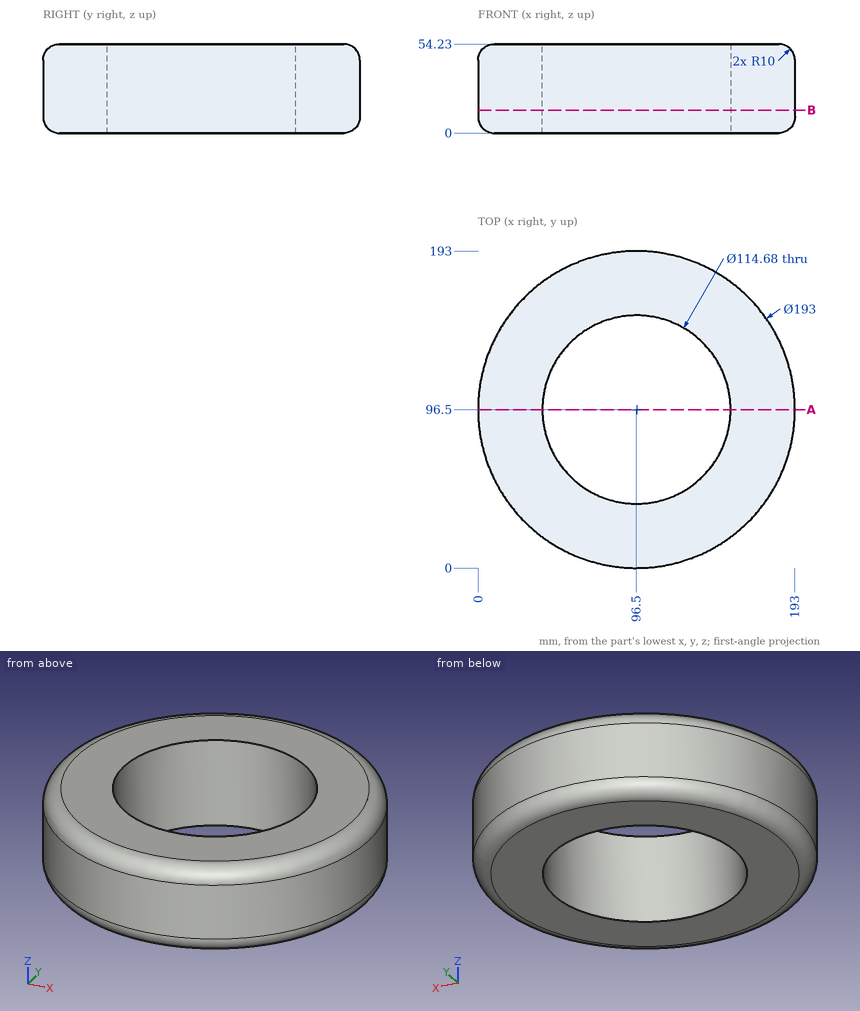
Part print with two shaded views. Sizes in mm from the minimum x, y, z corner. Round coordinates to 2 decimals unless told otherwise and drop trailing zeros. Order: outer loops, then holes, each group sorted by start corner. A loop starts at its lowest first (then second) coordinate and runs counter-clockwise, first axis right, second up.
(1) Band-saw the part on A-A (y = 96.5). List the corners of the cut face in (x, z), then the cut area to 3 significant figures.
(2) Band-saw the part on B-B (z = 14). List the corners of the cut face in (x, y).
(3) Pin check, flat tips, straight feed: pin 1 (6 mm diameter, centred on x = 150, y = 21, fed in from +Z); pin 2 (10 mm diameter, centred on x = 131, z = 20, fed in from -Y); pin 3 (10 mm diameter, centred on x = 107.5, z = 42.5, fed in from +Y). Stop position of each tip, or through.
(4) Drill centre lines: line 1 (X direction, y = 97.5, z = 10); line 2 (Y direction, x = 96, z = 34); line 3 (Y direction, x = 70, z = 19). Where is each one in solid material? Low to high.
Verdict:
1. outline: (0, 10) arc R10 ccw to (10, 0) - (39.16, 0) - (39.16, 54.23) - (10, 54.23) arc R10 ccw to (0, 44.23) - close; (153.84, 0) - (183, 0) arc R10 ccw to (193, 10) - (193, 44.23) arc R10 ccw to (183, 54.23) - (153.84, 54.23) - close
1. area: 4,160 mm2
2. outline: circle Ø193 at (96.5, 96.5); hole circle Ø114.68 at (96.5, 96.5)
3. pin 1: stops at z = 53.76
3. pin 2: stops at y = 4.62
3. pin 3: stops at y = 192.81
4. line 1: x = 0.01 to 39.17, 153.83 to 192.99
4. line 2: y = 0 to 39.16, 153.84 to 193
4. line 3: y = 3.71 to 45.65, 147.35 to 189.29
